Autodesk Inventor part; units mm, degrees
ref_plane "YZ Plane" through (0, 0, 0) normal (1, 0, 0) x (0, 1, 0)
ref_plane "XZ Plane" through (0, 0, 0) normal (0, 1, 0) x (-1, 0, 0)
ref_plane "XY Plane" through (0, 0, 0) normal (0, 0, 1) x (1, 0, 0)
sketch "Sketch1" plane through (0, 0, 0) normal (0, 1, 0) x (-1, 0, 0)
  line L0 (-200, 200) -> (200, 200)
  line L1 (200, 200) -> (200, -200)
  line L2 (200, -200) -> (-200, -200)
  line L3 (-200, -200) -> (-200, 200)
  line L4 (-200, 200) -> (200, -200) construction
  line L5 (200, 200) -> (-200, -200) construction
  point P0 (0, 0)
  dimension "d0" = 400
  dimension "d1" = 400
extrude "Extrusion1" add sketch "Sketch1" along normal blind 6
sketch "Sketch2" plane through (0, 6, 0) normal (0, 1, 0) x (1, 0, 0)
  line L0 (-190, -5) -> (-137.7238, -5)
  line L1 (-137.7238, -5) -> (-137.7238, 37.4)
  line L2 (-190, 37.4) -> (-137.7238, 37.4)
  line L3 (-190, -5) -> (-190, 37.4)
  line L4 (-142.7238, 32.4) -> (-142.7238, 0)
  line L5 (-142.7238, 0) -> (-185, 0)
  line L6 (-185, 0) -> (-185, 32.4)
  line L7 (-185, 32.4) -> (-142.7238, 32.4)
  line L8 (-127.7238, 47.4) -> (-127.7238, -15)
  line L9 (-127.7238, -15) -> (-200, -15)
  line L10 (-200, -15) -> (-200, 47.4)
  line L11 (-200, 47.4) -> (-127.7238, 47.4)
  line L12 (-132.7238, 42.4) -> (-132.7238, -10) construction
  line L13 (-132.7238, -10) -> (-195, -10) construction
  line L14 (-195, -10) -> (-195, 42.4) construction
  line L15 (-195, 42.4) -> (-132.7238, 42.4) construction
  circle A0 centre (-132.7238, 42.4) radius 2.5
  circle A1 centre (-195, 42.4) radius 2.5
  circle A2 centre (-195, -10) radius 2.5
  circle A3 centre (-132.7238, -10) radius 2.5
  line L16 (-200, -200) -> (200, -200)
  line L17 (-200, 200) -> (-200, -200)
  point P0 (0, 0)
  point P1 (-163.8619, -15)
  dimension "d4" = 5
  dimension "d5" = 10
  dimension "d6" = 5
  dimension "d7" = 5
  dimension "d8" = 5
  dimension "d9" = 5
  dimension "d10" = 5
  dimension "d11" = 62.4
  dimension "d12" = 72.2762
  dimension "d13" = 42.4
  dimension "d14" = 52.2762
  dimension "d18" = 185
extrude "Extrusion2" cut sketch "Sketch2" against normal through all contours L4 L5 L6 L7 | A0 | A1 | A2 | A3
sketch "Sketch3" plane through (0, 6, 0) normal (0, 1, 0) x (1, 0, 0)
  line L0 (200, 200) -> (-200, 200)
  line L1 (-200, 200) -> (-200, 320)
  line L2 (-200, 320) -> (-40, 320)
  line L3 (-40, 320) -> (-40, 200)
  line L4 (-180, 300) -> (-60, 300)
  line L5 (-60, 300) -> (-60, 220)
  line L6 (-60, 220) -> (-180, 220)
  line L7 (-180, 220) -> (-180, 300)
  point P0 (0, 0)
  point P1 (-120, 300)
  dimension "d19" = 120
  dimension "d20" = 160
  dimension "d21" = 120
  dimension "d22" = 80
  dimension "d23" = 20
  dimension "d24" = 20
extrude "Extrusion3" add sketch "Sketch3" against normal blind 6
sketch "Sketch4" plane through (0, 6, 0) normal (0, 1, 0) x (1, 0, 0)
  line L0 (-180, 210) -> (-60, 210)
  line L1 (-60, 210) -> (-60, 204)
  line L2 (-60, 204) -> (-180, 204)
  line L3 (-180, 204) -> (-180, 210)
  line L4 (-60, 220) -> (-180, 220)
  line L5 (-200, 320) -> (-200, -200)
  line L6 (-177, 210) -> (-177, 204)
  line L7 (-171, 210) -> (-171, 204)
  line L8 (-171, 210) -> (-171, 204)
  line L9 (-165, 210) -> (-165, 204)
  line L10 (-165, 210) -> (-165, 204)
  line L11 (-159, 210) -> (-159, 204)
  line L12 (-159, 210) -> (-159, 204)
  line L13 (-153, 210) -> (-153, 204)
  line L14 (-153, 210) -> (-153, 204)
  line L15 (-147, 210) -> (-147, 204)
  line L16 (-147, 210) -> (-147, 204)
  line L17 (-141, 210) -> (-141, 204)
  line L18 (-141, 210) -> (-141, 204)
  line L19 (-135, 210) -> (-135, 204)
  line L20 (-135, 210) -> (-135, 204)
  line L21 (-129, 210) -> (-129, 204)
  line L22 (-129, 210) -> (-129, 204)
  line L23 (-123, 210) -> (-123, 204)
  line L24 (-123, 210) -> (-123, 204)
  line L25 (-117, 210) -> (-117, 204)
  line L26 (-117, 210) -> (-117, 204)
  line L27 (-111, 210) -> (-111, 204)
  line L28 (-111, 210) -> (-111, 204)
  line L29 (-105, 210) -> (-105, 204)
  line L30 (-105, 210) -> (-105, 204)
  line L31 (-99, 210) -> (-99, 204)
  line L32 (-99, 210) -> (-99, 204)
  line L33 (-93, 210) -> (-93, 204)
  line L34 (-93, 210) -> (-93, 204)
  line L35 (-87, 210) -> (-87, 204)
  line L36 (-87, 210) -> (-87, 204)
  line L37 (-81, 210) -> (-81, 204)
  line L38 (-81, 210) -> (-81, 204)
  line L39 (-75, 210) -> (-75, 204)
  line L40 (-75, 210) -> (-75, 204)
  line L41 (-69, 210) -> (-69, 204)
  line L42 (-69, 210) -> (-69, 204)
  line L43 (-63, 210) -> (-63, 204)
  line L44 (-180, 220) -> (-180, 300)
  line L45 (-180, 300) -> (-60, 300)
  line L46 (-60, 300) -> (-60, 220)
  line L47 (-180, 260) -> (-60, 260) construction
  line L48 (-180, 310) -> (-60, 310)
  line L49 (-60, 310) -> (-60, 316)
  line L50 (-60, 316) -> (-180, 316)
  line L51 (-180, 316) -> (-180, 310)
  line L52 (-177, 310) -> (-177, 316)
  line L53 (-171, 310) -> (-171, 316)
  line L54 (-171, 310) -> (-171, 316)
  line L55 (-165, 310) -> (-165, 316)
  line L56 (-165, 310) -> (-165, 316)
  line L57 (-159, 310) -> (-159, 316)
  line L58 (-159, 310) -> (-159, 316)
  line L59 (-153, 310) -> (-153, 316)
  line L60 (-153, 310) -> (-153, 316)
  line L61 (-147, 310) -> (-147, 316)
  line L62 (-147, 310) -> (-147, 316)
  line L63 (-141, 310) -> (-141, 316)
  line L64 (-141, 310) -> (-141, 316)
  line L65 (-135, 310) -> (-135, 316)
  line L66 (-135, 310) -> (-135, 316)
  line L67 (-129, 310) -> (-129, 316)
  line L68 (-129, 310) -> (-129, 316)
  line L69 (-123, 310) -> (-123, 316)
  line L70 (-123, 310) -> (-123, 316)
  line L71 (-117, 310) -> (-117, 316)
  line L72 (-117, 310) -> (-117, 316)
  line L73 (-111, 310) -> (-111, 316)
  line L74 (-111, 310) -> (-111, 316)
  line L75 (-105, 310) -> (-105, 316)
  line L76 (-105, 310) -> (-105, 316)
  line L77 (-99, 310) -> (-99, 316)
  line L78 (-99, 310) -> (-99, 316)
  line L79 (-93, 310) -> (-93, 316)
  line L80 (-93, 310) -> (-93, 316)
  line L81 (-87, 310) -> (-87, 316)
  line L82 (-87, 310) -> (-87, 316)
  line L83 (-81, 310) -> (-81, 316)
  line L84 (-81, 310) -> (-81, 316)
  line L85 (-75, 310) -> (-75, 316)
  line L86 (-75, 310) -> (-75, 316)
  line L87 (-69, 310) -> (-69, 316)
  line L88 (-69, 310) -> (-69, 316)
  line L89 (-63, 310) -> (-63, 316)
  point P0 (0, 0)
  point P1 (-180, 207)
  point P2 (-177, 207)
  point P3 (-171, 207)
  point P4 (-165, 207)
  point P5 (-159, 207)
  point P6 (-153, 207)
  point P7 (-147, 207)
  point P8 (-141, 207)
  point P9 (-135, 207)
  point P10 (-129, 207)
  point P11 (-123, 207)
  point P12 (-117, 207)
  point P13 (-111, 207)
  point P14 (-105, 207)
  point P15 (-99, 207)
  point P16 (-93, 207)
  point P17 (-87, 207)
  point P18 (-81, 207)
  point P19 (-75, 207)
  point P20 (-69, 207)
  point P21 (-180, 313)
  point P22 (-177, 313)
  point P23 (-171, 313)
  point P24 (-165, 313)
  point P25 (-159, 313)
  point P26 (-153, 313)
  point P27 (-147, 313)
  point P28 (-141, 313)
  point P29 (-135, 313)
  point P30 (-129, 313)
  point P31 (-123, 313)
  point P32 (-117, 313)
  point P33 (-111, 313)
  point P34 (-105, 313)
  point P35 (-99, 313)
  point P36 (-93, 313)
  point P37 (-87, 313)
  point P38 (-81, 313)
  point P39 (-75, 313)
  point P40 (-69, 313)
  dimension "d27" = 120
  dimension "d28" = 6
  dimension "d29" = 10
  dimension "d30" = 20
  dimension "d31" = 3
  dimension "d32" = 6
  dimension "d35" = 6
extrude "Extrusion4" cut sketch "Sketch4" against normal blind 6 contours L0 L7 L2 L6 | L0 L11 L2 L9 | L0 L15 L2 L13 | L0 L19 L2 L17 | L0 L23 L2 L21 | L0 L27 L2 L25 | L0 L31 L2 L29 | L0 L35 L2 L33 | L0 L39 L2 L37 | L0 L43 L2 L41 | L52 L50 L53 L48 | L55 L50 L57 L48 | L59 L50 L61 L48 | L63 L50 L65 L48 | L67 L50 L69 L48 | L71 L50 L73 L48 | L75 L50 L77 L48 | L79 L50 L81 L48 | L83 L50 L85 L48 | L87 L50 L89 L48
sketch "Sketch5" plane through (0, 6, 0) normal (0, 1, 0) x (1, 0, 0)
  line L0 (200, -200) -> (200, 200)
  line L1 (200, 200) -> (-40, 200)
  line L2 (200, 0) -> (-40, 0)
  line L3 (-40, 0) -> (-40, 200)
  line L4 (-40, 200) -> (200, 200)
  line L5 (200, 200) -> (200, 0)
  point P0 (0, 0)
  dimension "d42" = 240
equation "\"d40\" = d32"
properties part number "base zzzz"
Model file for the job. Use its own axes, mm. Coordinates: 2 decimals unless noted, no trailing zeros. Order: outer loops, then holes, each group sorted by start corner. A loop starts at its lowest first (then second) coordinate and runs counter-clockwise, first axis right, second up. Notation, with made-up numbers: M 3.25,-8.75 L 54.25,-8.75 A17 ccw 54.25,22.25 Z; hole C 71,-29.75 d1. An arc over 180 degrees is marked long. Return JSON: item names as keys, results as strings.
1. Saw through at A-A (y = 2.5). Give the number of separate pieces and of enclosed holes in the cut face, and give its area (3 significant figures).
Ans:
{"separate pieces": "1", "enclosed holes": "26", "area": "167,000 mm^2"}
2. Drill centre lines: probe 1 along Z at (x, y) = (-195, 2.2); probe 2 along X at (y, z) = (3.05, -42.4); probe 3 along X at (y, z) = (3.55, -276). Where is each one in solid material? Low to high.
Ans:
{"probe 1": "-320 to -44.9, -39.9 to 7.5, 12.5 to 200", "probe 2": "-200 to -197.5, -192.5 to -135.22, -130.22 to 200", "probe 3": "-200 to -180, -60 to -40"}
3. Saw through at B-B (x = -28.5). Give the cut face in (y, z), and give its area (3 significant figures).
Ans:
{"outline": "M 0,-200 L 6,-200 L 6,200 L 0,200 Z", "area": "2,400 mm^2"}
4. Flat gauge pins, fed straight in: pin 1 (1.5 mm diameter, centred on y = 2, z = -258, fed in from +X); pin 2 (4 mm diameter, centred on x = -132.72, z = -42.4, fed in from +Y). Where does each tip first touch, or does it go through?
Ans:
{"pin 1": "x = -40", "pin 2": "through"}
